Geometry check sheet. Reference: the model listing, model coordinates, mm. A direction names the side the tool comes from. Coordinates: 2 decimals unless noted, no trailing zeros. Loops run counter-clockwise (first coordinate to the right, second up) from the corner with the lowest first, then second, coordinate; pieces in that order, holes last.
from build123d import *

# Parameters (mm, degrees)
SKETCH_1_W          = 15
SKETCH_1_H          = 10
EXTRUDE_1_DEPTH     = 3
SKETCH_2_W          = 3
SKETCH_2_H          = 10
EXTRUDE_2_DEPTH     = 12
SKETCH_3_R          = 1.5
CUT_EXTRUDE_1_DEPTH = 7
SKETCH_4_R          = 1.5
CUT_EXTRUDE_2_DEPTH = 7


with BuildPart() as part:
    # 草图1 → 凸台-拉伸1 (new body)
    with BuildSketch(Plane.XY):
        Rectangle(SKETCH_1_W, SKETCH_1_H)
    extrude(amount=EXTRUDE_1_DEPTH)

    # 草图2 → 凸台-拉伸2 (add)
    with BuildSketch(Plane.XY.offset(3)):
        with Locations((-6, 0)):
            Rectangle(SKETCH_2_W, SKETCH_2_H)
    extrude(amount=EXTRUDE_2_DEPTH)

    # 草图3 → 切除-拉伸1 (cut)
    with BuildSketch(Plane(origin=(0, 0, 0), x_dir=(-1, 0, 0), z_dir=(0, 0, -1))):
        Circle(SKETCH_3_R)
    extrude(amount=-CUT_EXTRUDE_1_DEPTH, mode=Mode.SUBTRACT)

    # 草图4 → 切除-拉伸2 (cut)
    with BuildSketch(Plane.ZY.offset(7.5)):
        with Locations((7.5, 0)):
            Circle(SKETCH_4_R)
    extrude(amount=-CUT_EXTRUDE_2_DEPTH, mode=Mode.SUBTRACT)


solid = part.part
1) Depth check by flat-ended pin: pin 1 (1.5 mm diameter, centred on x = -5, y = -1, fed in from -Z); pin 2 (3 mm diameter, centred on x = 3.5, y = -2.5, fed in from +Z); pin 3 (2.5 mm diameter, centred on x = 0, y = 0, fed in from -Z). Enter the tip coordinate at first touch or a pass-through.
Data:
pin 1: stops at z = 0
pin 2: stops at z = 3
pin 3: passes through
2) Section check D-D on z = 2. Record the cut outline in (x, y), and give its area (3 significant figures).
Data:
outline: (-7.5, -5) - (7.5, -5) - (7.5, 5) - (-7.5, 5) - close; hole circle Ø3 at (0, 0)
area: 143 mm2
3) Section check C-C on z = 7.5. Record the cut outline in (x, y).
Data:
outline: (-7.5, -5) - (-4.5, -5) - (-4.5, -1.5) - (-7.5, -1.5) - close; (-7.5, 1.5) - (-4.5, 1.5) - (-4.5, 5) - (-7.5, 5) - close
4) Section check A-A on x = 0. Record the cut outline in (y, z), and give its area (3 significant figures).
Data:
outline: (-5, 0) - (-1.5, 0) - (-1.5, 3) - (-5, 3) - close; (1.5, 0) - (5, 0) - (5, 3) - (1.5, 3) - close
area: 21.0 mm2
5) Access from +Z, -Z, +X, -X, +Y, -Y to the whole of each face (thin tool, end or side, straight path). Record for faces 1 (the flat face through (-4.5, -1, 9)), 2 (the cylindrical face through (1.5, 0.07, 1.48)).
Data:
face 1: +Z, +X, +Y, -Y
face 2: +Z, -Z
6) Material ranges on probe 1 along Y at (x, z) = (-6.05, 7.5); probe 2 along X at (y, z) = (-3.5, 13); probe 3 along Z at (x, y) = (4.5, 2), recorded low to high.
Data:
probe 1: y = -5 to -1.5, 1.5 to 5
probe 2: x = -7.5 to -4.5
probe 3: z = 0 to 3
7) Mould release check, pull along Z, two halves, no side actions. Record for faces 3 (the cylindrical face through (-6, 0, 6)), 4 (the flat face through (-7.5, -0.1, 5.7)), 5 (the flat face through (-2, 0, 0)): +Z half, -Z half, draft (parallel to the pull), parting line (faces both ways), or undercut.
Data:
face 3: undercut
face 4: draft
face 5: -Z half
8) Section check B-B on y = 0. Record the cut outline in (x, z), and give its area (3 significant figures).
Data:
outline: (-7.5, 0) - (-1.5, 0) - (-1.5, 3) - (-4.5, 3) - (-4.5, 6) - (-7.5, 6) - close; (-7.5, 9) - (-4.5, 9) - (-4.5, 15) - (-7.5, 15) - close; (1.5, 0) - (7.5, 0) - (7.5, 3) - (1.5, 3) - close
area: 63.0 mm2
